from build123d import *

# Parameters (mm, degrees)
SKETCH1_R           = 1.27
BOSS_EXTRUDE2_DEPTH = 1.5875
SKETCH2_W           = 15.24
SKETCH2_H           = 1.5875
BOSS_EXTRUDE3_DEPTH = 48.26
SKETCH3_R           = 1
CUT_EXTRUDE1_DEPTH  = 2.54
SKETCH4_R           = 1
CUT_EXTRUDE2_DEPTH  = 2.54
SKETCH5_R           = 1
CUT_EXTRUDE3_DEPTH  = 2.54
SKETCH6_W           = 2.032
SKETCH6_H           = 7.366
CUT_EXTRUDE4_DEPTH  = 2.54


with BuildPart() as part:
    # Sketch1 → Boss-Extrude2 (new body)
    with BuildSketch(Plane(origin=(0, 0, 0), x_dir=(1, 0, 0), z_dir=(0, 1, 0))):
        with BuildLine():
            Line((50.8, 0), (50.8, 11.43))
            Line((50.8, 11.43), (43.18, 24.628227154))
            Line((43.18, 24.628227154), (30.9, 24.628227154))
            Line((30.9, 24.628227154), (30.9, 18.264121265))
            ThreePointArc((30.9, 18.264121265), (25.4, 12.764121265), (19.9, 18.264121265))
            Line((19.9, 18.264121265), (19.9, 24.628227154))
            Line((19.9, 24.628227154), (7.62, 24.628227154))
            Line((7.62, 24.628227154), (0, 11.43))
            Line((0, 11.43), (0, 0))
            Line((0, 0), (17.78, 0))
            Line((17.78, 0), (17.78, -19.327878735))
            Line((17.78, -19.327878735), (33.02, -19.327878735))
            Line((33.02, -19.327878735), (33.02, 0))
            Line((33.02, 0), (50.8, 0))
        make_face()
        with Locations(Location((14.401477372, 11.914121265, 0), (0, 0, 270))):
            Circle(SKETCH1_R, mode=Mode.SUBTRACT)
        with Locations(Location((36.398522628, 11.914121265, 0), (0, 0, 270))):
            Circle(SKETCH1_R, mode=Mode.SUBTRACT)
        with Locations(Location((10.409113577, 14.219113577, 0), (0, 0, 270))):
            Circle(SKETCH1_R, mode=Mode.SUBTRACT)
        with Locations(Location((40.390886423, 14.219113577, 0), (0, 0, 270))):
            Circle(SKETCH1_R, mode=Mode.SUBTRACT)
        with Locations(Location((43.690443212, 16.124113577, 0), (0, 0, 270))):
            Circle(SKETCH1_R, mode=Mode.SUBTRACT)
        with Locations(Location((7.109556788, 16.124113577, 0), (0, 0, 270))):
            Circle(SKETCH1_R, mode=Mode.SUBTRACT)
        with Locations(Location((25.4, -7.135878735, 0), (0, 0, 270))):
            Circle(SKETCH1_R, mode=Mode.SUBTRACT)
        with Locations(Location((25.4, -15.517878735, 0), (0, 0, 270))):
            Circle(SKETCH1_R, mode=Mode.SUBTRACT)
        with Locations(Location((25.4, -11.707878735, 0), (0, 0, 270))):
            Circle(SKETCH1_R, mode=Mode.SUBTRACT)
    extrude(amount=BOSS_EXTRUDE2_DEPTH)

    # Sketch2 → Boss-Extrude3 (add)
    with BuildSketch(Plane(origin=(0, 1.5875, 0), x_dir=(1, 0, 0), z_dir=(0, 1, 0))):
        with Locations((25.4, -18.534128735)):
            Rectangle(SKETCH2_W, SKETCH2_H)
        Polygon((0, 11.43), (7.62, 24.628227154), (8.994815329, 23.834477154), (1.374815329, 10.63625), align=None)
        Polygon((50.8, 11.43), (43.18, 24.628227154), (41.806418442, 23.835189471), (49.460038325, 10.578730971), align=None)
    extrude(amount=BOSS_EXTRUDE3_DEPTH)

    # Sketch3 → Cut-Extrude1 (cut)
    with BuildSketch(Plane.XY.offset(19.327878735)):
        with Locations((25.4, 42.1025)):
            Circle(SKETCH3_R)
        with Locations((25.4, 29.4025)):
            Circle(SKETCH3_R)
    extrude(amount=-CUT_EXTRUDE1_DEPTH, mode=Mode.SUBTRACT)

    # Sketch4 → Cut-Extrude2 (cut)
    with BuildSketch(Plane(origin=(43.049335183, 0, -24.854545256), x_dir=(-0.5000000000000016, 0, -0.8660254037844378), z_dir=(0.8660254037844378, 0, -0.5000000000000016))):
        with Locations((-7.881329635, 42.1025)):
            Circle(SKETCH4_R)
        with Locations((-7.881329635, 29.4025)):
            Circle(SKETCH4_R)
    extrude(amount=-CUT_EXTRUDE2_DEPTH, mode=Mode.SUBTRACT)

    # Sketch5 → Cut-Extrude3 (cut)
    with BuildSketch(Plane(origin=(-4.949335183, 0, -2.8575), x_dir=(-0.5000000000000012, 0, 0.866025403784438), z_dir=(-0.8660254037844379, 0, -0.5000000000000011))):
        with Locations((-17.334430776, 42.104691674)):
            Circle(SKETCH5_R)
        with Locations((-17.334430776, 29.404691674)):
            Circle(SKETCH5_R)
    extrude(amount=-CUT_EXTRUDE3_DEPTH, mode=Mode.SUBTRACT)

    # Sketch6 → Cut-Extrude4 (cut)
    with BuildSketch(Plane(origin=(0, 0, 0), x_dir=(-1, 0, 0), z_dir=(0, -1, 0))):
        with Locations((-18.796, -7.008878735)):
            Rectangle(SKETCH6_W, SKETCH6_H)
    extrude(amount=-CUT_EXTRUDE4_DEPTH, mode=Mode.SUBTRACT)


solid = part.part
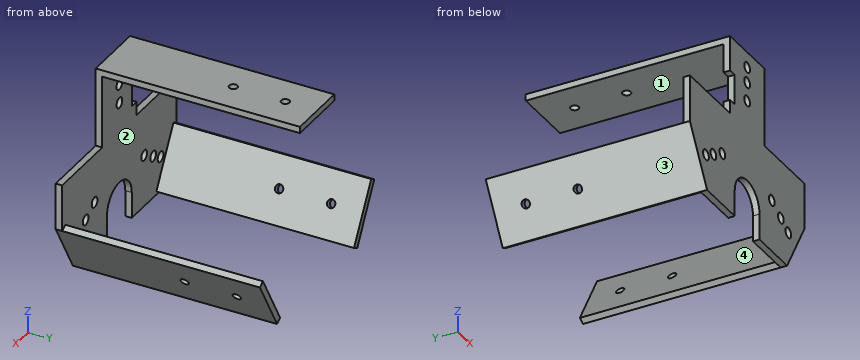
Source: CAD feature listing. Evaluate the final solid. Frame: model axes, mm. Face numbers are marked on the shaded views. A direction names the side the tool comes from. Round coordinates to 2 decimals unless told otherwise and drop trailing zeros. Loops run counter-clockwise (first coordinate to the right, second up) from the corner with the lowest first, then second, coordinate; pieces in that order, holes last. Notation, with made-up numbers: M 29.25,-40 L 45.25,-40 A29 ccw 45.25,-12 Z; hole C 73.25,73 d5. An arc over 180 degrees is marked long. Return JSON: item names as keys, results as strings. Group by question number.
1. Section query A-A on y = 45.5. Output: boundary loops of the cut face in (x, z), and give its area (3 significant figures).
2. Reachability of the marked faces 1, 2, 3 and 4 from +Z, -Z, +X, -X, +Y, -Y: full face, straight path, thin tool, end or side. Return the list, or none.
3. Material intervals for line 1 along Y through (x, z) = (25.4, 18.55); line 2 along X through (y, z) = (37.5, -18); line 3 along Z through (x, y) = (24, 43.5), sorted ascending. Write a range as from..to.
4. Section query D-D on z = -4. Output: boundary loops of the cut face in (x, y), and give its area (3 significant figures).
5. Pin query (flat end, axial travel): pin 1 (2.5 mm diameter, centred on x = 25.4, y = 42.1, fed in from -Z); pin 2 (3 mm diameter, centred on x = 34, z = -12, fed in from +Y); pin 3 (1.5 mm diameter, centred on x = 42, y = 33.5, fed in from +Z); pin 4 (2 mm diameter, centred on x = 43.69, z = -16.12, fed in from -Y). Return the tip coordinate at first contact, or that it passes through.
6. Section query C-C on z = 7. Output: boundary loops of the cut face in (x, y), and give its area (3 significant figures).
7. Section query B-B on x = 25.4. Output: boundary loops of the cut face in (y, z), and give its area (3 significant figures).
Checks:
{
 "1": {"outline": "M 0,-11.43 L 7.62,-24.63 L 8.99,-23.83 L 1.37,-10.64 Z; M 17.78,17.74 L 33.02,17.74 L 33.02,19.33 L 17.78,19.33 Z; M 41.81,-23.84 L 43.18,-24.63 L 50.8,-11.43 L 49.46,-10.58 Z", "area": "72.6 mm²"},
 "2": {"face 1": "-Z, +X, -X, +Y", "face 2": "+Y", "face 3": "-Z, -X, +Y, -Y", "face 4": "+Z, +Y"},
 "3": {"line 1": "y = 0..28.4, 30.4..41.1, 43.1..49.85", "line 2": "x = 3.79..5.63, 45.18..47.01", "line 3": "z = 17.74..19.33"},
 "4": {"outline": "M 0,0 L 50.8,0 L 50.8,1.59 L 0,1.59 Z", "area": "80.6 mm²"},
 "5": {"pin 1": "stops at z = 17.74", "pin 2": "stops at y = 1.59", "pin 3": "stops at z = -22.2", "pin 4": "passes through"},
 "6": {"outline": "M 19.81,0 L 24.14,0 L 24.14,1.59 L 19.81,1.59 Z; M 26.66,0 L 33.02,0 L 33.02,1.59 L 26.66,1.59 Z", "area": "17.0 mm²"},
 "7": {"outline": "M 0,-12.76 L 1.59,-12.76 L 1.59,5.87 L 0,5.87 Z; M 0,8.41 L 1.59,8.41 L 1.59,10.44 L 0,10.44 Z; M 0,12.98 L 1.59,12.98 L 1.59,14.25 L 0,14.25 Z; M 0,16.79 L 1.59,16.79 L 1.59,17.74 L 28.4,17.74 L 28.4,19.33 L 0,19.33 Z; M 30.4,17.74 L 41.1,17.74 L 41.1,19.33 L 30.4,19.33 Z; M 43.1,17.74 L 49.85,17.74 L 49.85,19.33 L 43.1,19.33 Z", "area": "109 mm²"}
}
